Design review of the part built by this model. Coordinates are the model's own, in mm. A direction names the side the tool comes from. Coordinates: 2 decimals unless noted, no trailing zeros. Write each loop counter-clockwise with the first axis right and the second up, starting at its lowest first coordinate (ties: lowest second). Pieces come first, ordered by that corner, then holes. Notation, with made-up numbers: M -0.75,84 L 51.25,84 A12 cw 51.25,103 Z; hole C 67.25,49 d6. An arc over 180 degrees is marked long. Write each question's results on one line, items separated by ' | '. Start each with the question number.
```python
from build123d import *

# Parameters (mm, degrees)
SKETCH_1_W          = 30
SKETCH_1_H          = 15
EXTRUDE_1_DEPTH     = 1.5
SKETCH_2_W          = 4
SKETCH_2_H          = 9.5
EXTRUDE_2_DEPTH     = 10
SKETCH_3_R          = 1.15
EXTRUDE_3_DEPTH     = 1.8
SKETCH_5_W          = 2.5
SKETCH_5_H          = 2
EXTRUDE_4_DEPTH     = 2.5
CHAMFER_1_SIZE      = 0.2
SKETCH_6_W          = 2.1
SKETCH_6_H          = 0.2
EXTRUDE_5_DEPTH     = 2
SKETCH_7_W          = 0.5
SKETCH_7_H          = 0.5
EXTRUDE_6_DEPTH     = 1.8
SKETCH_8_W          = 0.5
SKETCH_8_H          = 0.5
EXTRUDE_7_DEPTH     = 6.7
FILLET_1_R          = 0.5
SKETCH_10_R         = 0.747999162
CUT_EXTRUDE_1_DEPTH = 39.294647146
SKETCH_11_W         = 5
SKETCH_11_H         = 3.4
EXTRUDE_8_DEPTH     = 1.5
SKETCH_12_W         = 2.7
SKETCH_12_H         = 1.2
EXTRUDE_9_DEPTH     = 0.6
SKETCH_13_W         = 1.6
SKETCH_13_H         = 1.3
EXTRUDE_10_DEPTH    = 1
SKETCH_14_W         = 1
SKETCH_14_H         = 1
EXTRUDE_11_DEPTH    = 0.2
SKETCH_15_W         = 2.2
SKETCH_15_H         = 1.2
EXTRUDE_12_DEPTH    = 0.6
SKETCH_17_R         = 0.5
CUT_EXTRUDE_2_DEPTH = 39.294647146
SKETCH_18_W         = 0.5
SKETCH_18_H         = 0.5
EXTRUDE_13_DEPTH    = 9
SKETCH_20_W         = 2
SKETCH_20_H         = 4
EXTRUDE_14_DEPTH    = 3
CHAMFER_2_SIZE      = 0.5


with BuildPart() as part:
    # 草图1 → 凸台-拉伸1 (new body)
    with BuildSketch(Plane.XY):
        with Locations((15, 7.5)):
            Rectangle(SKETCH_1_W, SKETCH_1_H)
    extrude(amount=EXTRUDE_1_DEPTH)

    # 草图2 → 凸台-拉伸2 (add)
    with BuildSketch(Plane.XY.offset(1.5)):
        with Locations((19, 5.75)):
            Rectangle(SKETCH_2_W, SKETCH_2_H)
    extrude(amount=EXTRUDE_2_DEPTH)

    # 草图3 → 凸台-拉伸3 (add)
    with BuildSketch(Plane.XY.offset(11.5)):
        with Locations((19.85, 9.35)):
            Circle(SKETCH_3_R)
    extrude(amount=EXTRUDE_3_DEPTH)

    # 草图5 → 凸台-拉伸4 (add)
    with BuildSketch(Plane.XY.offset(1.5)):
        with Locations((26.25, 10)):
            Rectangle(SKETCH_5_W, SKETCH_5_H)
        with Locations((26.25, 7.8)):
            Rectangle(SKETCH_5_W, SKETCH_5_H)
        with Locations((26.25, 5.6)):
            Rectangle(SKETCH_5_W, SKETCH_5_H)
    extrude(amount=EXTRUDE_4_DEPTH)

    # 倒角1
    chamfer_1_edges = [part.edges().sort_by_distance(p)[0] for p in [
        (25, 11, 2.75),
        (25, 9, 2.75),
        (27.5, 9, 2.75),
        (27.5, 11, 2.75),
        (27.5, 8.8, 2.75),
        (25, 8.8, 2.75),
        (25, 6.8, 2.75),
        (27.5, 6.8, 2.75),
        (27.5, 6.6, 2.75),
        (25, 6.6, 2.75),
        (25, 4.6, 2.75),
        (27.5, 4.6, 2.75),
    ]]
    chamfer(chamfer_1_edges, length=CHAMFER_1_SIZE)

    # 草图6 → 凸台-拉伸5 (add)
    with BuildSketch(Plane.XY.offset(1.5)):
        with Locations((26.25, 8.9)):
            Rectangle(SKETCH_6_W, SKETCH_6_H)
        with Locations((26.25, 6.7)):
            Rectangle(SKETCH_6_W, SKETCH_6_H)
    extrude(amount=EXTRUDE_5_DEPTH)

    # 草图7 → 凸台-拉伸6 (add)
    with BuildSketch(Plane.XY.offset(4)):
        with Locations((26.25, 5.6)):
            Rectangle(SKETCH_7_W, SKETCH_7_H)
        with Locations((26.25, 7.8)):
            Rectangle(SKETCH_7_W, SKETCH_7_H)
        with Locations((26.25, 10)):
            Rectangle(SKETCH_7_W, SKETCH_7_H)
    extrude(amount=EXTRUDE_6_DEPTH)

    # 草图8 → 凸台-拉伸7 (add)
    with BuildSketch(Plane(origin=(26.5, 0, 0), x_dir=(0, 0, -1), z_dir=(1, 0, 0))):
        with Locations((-5.55, 5.6)):
            Rectangle(SKETCH_8_W, SKETCH_8_H)
        with Locations((-5.55, 7.8)):
            Rectangle(SKETCH_8_W, SKETCH_8_H)
        with Locations((-5.55, 10)):
            Rectangle(SKETCH_8_W, SKETCH_8_H)
    extrude(amount=EXTRUDE_7_DEPTH)

    # 圆角1
    fillet_1_edges = [part.edges().sort_by_distance(p)[0] for p in [
        (26, 5.6, 5.8),
        (26, 7.8, 5.8),
        (26, 10, 5.8),
        (26.5, 5.6, 5.3),
        (26.5, 7.8, 5.3),
        (26.5, 10, 5.3),
    ]]
    fillet(fillet_1_edges, radius=FILLET_1_R)

    # 草图10 → 切除-拉伸1 (cut, through all)
    with BuildSketch(Plane.XY.offset(1.5)):
        with Locations((23.5, 10)):
            Circle(SKETCH_10_R)
        with Locations((23.5, 7.8)):
            Circle(SKETCH_10_R)
        with Locations((23.5, 5.6)):
            Circle(SKETCH_10_R)
    extrude(amount=-CUT_EXTRUDE_1_DEPTH, mode=Mode.SUBTRACT)

    # 草图11 → 凸台-拉伸8 (add)
    with BuildSketch(Plane.XY.offset(1.5)):
        with Locations((13.5, 7.6)):
            Rectangle(SKETCH_11_W, SKETCH_11_H)
    extrude(amount=EXTRUDE_8_DEPTH)

    # 草图12 → 凸台-拉伸9 (add)
    with BuildSketch(Plane.XY.offset(1.5)):
        with Locations((12.35, 12.9)):
            Rectangle(SKETCH_12_W, SKETCH_12_H)
    extrude(amount=EXTRUDE_9_DEPTH)

    # 草图13 → 凸台-拉伸10 (add)
    with BuildSketch(Plane.XY.offset(1.5)):
        with Locations((11.8, 1.65)):
            Rectangle(SKETCH_13_W, SKETCH_13_H)
    extrude(amount=EXTRUDE_10_DEPTH)

    # 草图14 → 凸台-拉伸11 (add)
    with BuildSketch(Plane.XY.offset(1.5)):
        with Locations((7.5, 12.016968403)):
            Rectangle(SKETCH_14_W, SKETCH_14_H)
        with Locations((8.7, 12.016968403)):
            Rectangle(SKETCH_14_W, SKETCH_14_H)
        with Locations((8.7, 8.516968403)):
            Rectangle(SKETCH_14_W, SKETCH_14_H)
        with Locations((7.5, 8.516968403)):
            Rectangle(SKETCH_14_W, SKETCH_14_H)
    extrude(amount=EXTRUDE_11_DEPTH)

    # 草图15 → 凸台-拉伸12 (add)
    with BuildSketch(Plane.XY.offset(1.5)):
        with Locations((8.1, 5.1)):
            Rectangle(SKETCH_15_W, SKETCH_15_H)
        with Locations((8.1, 1.6)):
            Rectangle(SKETCH_15_W, SKETCH_15_H)
    extrude(amount=EXTRUDE_12_DEPTH)

    # 草图17 → 切除-拉伸2 (cut, through all)
    with BuildSketch(Plane.XY.offset(1.5)):
        with Locations((4, 9)):
            Circle(SKETCH_17_R)
    extrude(amount=-CUT_EXTRUDE_2_DEPTH, mode=Mode.SUBTRACT)

    # 草图18 → 凸台-拉伸13 (add)
    with BuildSketch(Plane.XY.offset(1.5)):
        with Locations((3.75, 5.75)):
            Rectangle(SKETCH_18_W, SKETCH_18_H)
        with Locations((1.75, 7.75)):
            Rectangle(SKETCH_18_W, SKETCH_18_H)
        with Locations((1.75, 5.75)):
            Rectangle(SKETCH_18_W, SKETCH_18_H)
    extrude(amount=EXTRUDE_13_DEPTH)

    # 草图20 → 凸台-拉伸14 (add)
    with BuildSketch(Plane.XY.offset(10.5)):
        with Locations((2.75, 6.75)):
            Rectangle(SKETCH_20_W, SKETCH_20_H)
    extrude(amount=EXTRUDE_14_DEPTH)

    # 倒角2
    chamfer_2_edges = [part.edges().sort_by_distance(p)[0] for p in [
        (1.75, 8.75, 12),
        (1.75, 4.75, 12),
    ]]
    chamfer(chamfer_2_edges, length=CHAMFER_2_SIZE)


solid = part.part
```
Item 1: We need section B-B on x = 13. State the section outline as (y, z) points.
Item 2: Wall thickness on L1, parallel to Y at x = 23.5, z = 0.9; L2, parallel to X at y = 1.5, z = 2; L3, parallel to Y at x = 4, z = 0.8: over which ranges is each line inside the solid? List them lowest first.
Item 3: We need section A-A on z = 10. State the section outline as (x, y) points, then the cut area to 4 significant figures.
Item 4: Insertion check: pin 1 Ø2 at (x, y) = (25.5, 6) entering from +Z; pin 2 Ø8 at (y, z) = (5, 6) entering from -X; pin 3 Ø4 at (x, z) = (24.5, 10) entering from +Y; pin 4 Ø1.7 at (x, y) = (13.5, 7.5) entering from +Z. Each pin has a flat end and moves straight along its axis. Give the tip position at first contact, or say it passes through.
Item 5: Draft analysis for pull direction X (two halves, no side actions). For faces 4 (the cylindrical face through (24.213, 5.825, 0.76)), 5 (the flat face through (28.7, 5.85, 5.5)), 6 (the cylindrical face through (3.892, 8.512, 0.76)), 7 (the flat face through (27.5, 10, 3)), state which applies: released by +X, released by -X, zero draft, split by the parting line, or undercut.
Item 6: For faces 1 (the flat face through (19, 1, 6)), 2 (the flat face through (8, 2, 2.1)), 3 (the flat face through (3, 4.75, 12)), list the 3-axis set-ups (+Z, -Z, +X, -X, +Y, -Y) from which the entire face can be reached by the end or side of a thin tool; tool diameter is ignored.
Answer:
1) outline: M 0,0 L 15,0 L 15,1.5 L 13.5,1.5 L 13.5,2.1 L 12.3,2.1 L 12.3,1.5 L 9.3,1.5 L 9.3,3 L 5.9,3 L 5.9,1.5 L 0,1.5 Z
2) L1: y = 0 to 4.85, 6.35 to 7.05, 8.55 to 9.25, 10.75 to 15 | L2: x = 7 to 9.2, 11 to 12.6, 17 to 21 | L3: y = 0 to 8.5, 9.5 to 15
3) outline: M 1.5,5.5 L 2,5.5 L 2,6 L 1.5,6 Z; M 1.5,7.5 L 2,7.5 L 2,8 L 1.5,8 Z; M 3.5,5.5 L 4,5.5 L 4,6 L 3.5,6 Z; M 17,1 L 21,1 L 21,10.5 L 17,10.5 Z | area: 38.75 mm^2
4) pin 1: stops at z = 5.8 | pin 2: stops at x = 1.5 | pin 3: passes through | pin 4: stops at z = 3
5) face 4: undercut | face 5: zero draft | face 6: undercut | face 7: released by +X
6) face 1: +Z, +X, -X, -Y | face 2: +Z, -X, +Y, -Y | face 3: +Z, -X, -Y
